Autodesk Inventor part; units mm, degrees
ref_plane "Work Plane1" through (-6.9215, -6.9215, 7.4676) normal (0, 0, -1) x (0, 1, 0)
ref_plane "YZ Plane" through (0, 0, 0) normal (1, 0, 0) x (0, 1, 0)
ref_plane "XZ Plane" through (0, 0, 0) normal (0, 1, 0) x (-1, 0, 0)
sketch "Sketch1" plane through (0, 0, 0) normal (0, 0, 1) x (1, 0, 0)
  circle A0 centre (0, 0) radius 6.477
  arc A1 (9.8184, 2.6122) -> (-9.8184, 2.6122) centre (0, 0) ccw
  line L0 (0, -10.16) -> (-20, -10.16)
  line L1 (-20, -10.16) -> (-20, -5.08)
  line L2 (0, -5.08) -> (0, -10.16)
  line L3 (0, -10.16) -> (20, -10.16)
  line L4 (20, -10.16) -> (20, -5.08)
  line L5 (0, -5.08) -> (0, -10.16)
  line L6 (-16, -5.08) -> (-16, -10.16) construction
  line L7 (-19.5, -5.08) -> (-19.5, -10.16) construction
  line L8 (-12.5, -5.08) -> (-12.5, -10.16) construction
  line L9 (-11.865, -5.08) -> (-11.865, -10.16) construction
  line L10 (-11.865, -5.08) -> (-9.8184, 2.6122)
  line L11 (16, -5.08) -> (16, -10.16) construction
  line L12 (12.5, -5.08) -> (12.5, -10.16) construction
  line L13 (11.865, -5.08) -> (11.865, -10.16) construction
  line L14 (11.865, -5.08) -> (9.8184, 2.6122)
  line L15 (20, -5.08) -> (11.865, -5.08)
  line L16 (-20, -5.08) -> (-11.865, -5.08)
  dimension "d0" = 12.954
  dimension "d1" = 20.32
  dimension "d3" = 5.08
  dimension "d5" = 5.08
  dimension "d6" = 16
  dimension "d7" = 3.5
  dimension "d8" = 3.5
  dimension "d9" = 0.635
  dimension "d10" = 16
  dimension "d11" = 3.5
  dimension "d12" = 0.635
ref_plane "Work Plane1" through (-6.9215, -6.9215, 7.4676) normal (0, 0, -1) x (0, 1, 0)
extrude "Extrusion1" add sketch "Sketch1" along normal up to surface (7.4676 mm away)
sketch "Sketch3" plane through (20, -10.16, 0) normal (1, 0, 0) x (0, 0, -1)
  line L0 (-7.4676, 5.08) -> (-7.4676, 0)
  line L1 (-7.4676, 0) -> (0, -2.5713)
  line L2 (-7.4676, 0) -> (0.6469, 0) construction
  line L3 (0, 0) -> (0, -2.5713)
  line L4 (0, 0) -> (-7.4676, 0)
  line L5 (0, 0) -> (-7.4676, 0)
  point P0 (0, 10.16)
  dimension "d28" = 19
extrude "Extrusion2" add sketch "Sketch3" against normal up to surface (40 mm away)
sketch "Sketch4" plane through (20, -5.08, 7.4676) normal (1, 0, 0) x (0, 0, -1)
  line L0 (7.4676, 0) -> (0, 0)
  line L1 (7.4676, 0) -> (0, 0)
  line L2 (7.4676, 0) -> (0, 2.5713)
  line L3 (0, 0) -> (0, 7.6922)
  line L4 (7.4676, 0) -> (15.3655, 0) construction
  line L5 (0, 7.6922) -> (0, 0)
  line L6 (0, 2.5713) -> (0, 0)
  point P0 (7.4676, 5.08)
  dimension "d31" = 161
extrude "Extrusion3" add sketch "Sketch4" against normal blind 10.16
sketch "Sketch5" plane through (-20, -5.08, 0) normal (-1, 0, 0) x (0, 0, 1)
  line L0 (7.4676, 7.6922) -> (7.4676, 0)
  line L1 (0, 0) -> (7.4676, 0)
  line L2 (0, 0) -> (7.4676, 2.5713)
  line L3 (0, 0) -> (7.8979, 0) construction
  line L4 (7.4676, 0) -> (7.4676, -5.08)
  line L5 (7.4676, 2.5713) -> (7.4676, 0)
  point P0 (0, 5.08)
  dimension "d34" = 19
extrude "Extrusion4" add sketch "Sketch5" against normal blind 10.16
sketch "Sketch6" plane through (-20, -12.7313, 0) normal (0, -0.9455, 0.3256) x (1, 0, 0)
  line L0 (40, 2.491) -> (40, 10.3889) construction
  line L1 (40, 3.8979) -> (0, 3.8979) construction
  line L2 (0, 7.8979) -> (40, 7.8979) construction
  line L3 (36, 7.8979) -> (36, 0) construction
  line L4 (40, 0) -> (0, 0) construction
  line L5 (40, 7.8979) -> (40, 0) construction
  line L6 (4, 7.8979) -> (4, 0) construction
  line L7 (0, 7.8979) -> (0, 0) construction
  circle A0 centre (36, 3.8979) radius 2.1844
  circle A1 centre (4, 3.8979) radius 2.1844
  point P0 (20, 4.1449)
  dimension "d37" = 4
  dimension "d38" = 4
  dimension "d39" = 4
  dimension "d40" = 4.3688
  dimension "d41" = 4.3688
hole "Hole2" at (16, -11.4623, 3.6855) at (-16, -11.4623, 3.6855) direction (0, 0.9455, -0.3256) diameter 4.3688 end through all
properties part number "omni wheel shaft holder low channel side attach"
Check sheet for the modelled part. Datum: model origin and axes. Units: mm. A direction names the side the tool comes from. Coordinates: 2 decimals unless noted, no trailing zeros. Loops run counter-clockwise (first coordinate to the right, second up) from the corner with the lowest first, then second, coordinate; pieces in that order, holes last.
1) Access from +Z, -Z, +X, -X, +Y, -Y to the whole of each face (thin tool, end or side, straight path). Record for faces 5 (the face through (0, -7, 7.468)), 6 (the face through (-10.629, -0.433, 3.682)), 7 (the face through (15.652, -3.527, 4.511)).
2) Sectioned sample at C-C (z = 6.75). Record the boundary of the cut face in (x, y).
3) Sectioned sample at D-D (z = 2). Count the separate pieces of the cut face and the enclosed holes in it, and give its area (3 significant figures).
4) Sectioned sample at B-B (y = -3.25). Record the boundary of the cut face in (x, z), and give its area (3 significant figures).
5) Release check for a two-part mould opening along Y. For faces 1 (the face through (-20, -8, 4)), 2 (the face through (-0.19, 10.16, 3.68)), 3 (the face through (0.28, -11.428, 3.786)), 4 (the face through (-16.096, -7.284, 4.555)) record: released by +Y, released by -Y, zero draft, split by the parting line, or undercut.
6) Gauge pin test, flat ends, axial feed: pin 1 (1 mm diameter, centred on x = -2, z = 3.5, fed in from +Y); pin 2 (3 mm diameter, centred on x = 7.5, z = 4, fed in from +Y). Record the tip position at first contact, or that the pin passes through.
7) Material ranges on probe 1 along Y at (x, z) = (-3, 6.25); probe 2 along X at (y, z) = (-5.5, 5); probe 3 along X at (y, z) = (4, 5.25), recorded low to high.
8) Sectioned sample at A-A (x = 0). Record the boundary of the cut face in (y, z).
Check sheet entries:
1. face 5: +Z, +X, -X, +Y, -Y
1. face 6: -Z, -X, +Y
1. face 7: -Z, +X, +Y
2. outline: (-20, -10.41) - (20, -10.41) - (20, -2.76) - (11.25, -2.76) - (9.82, 2.61) arc R10.16 ccw to (-9.82, 2.61) - (-11.25, -2.76) - (-20, -2.76) - close; hole circle Ø12.95 at (0, 0)
3. separate pieces: 3
3. enclosed holes: 1
3. area: 374 mm2
4. outline: (-20, 5.31) - (-11.38, 5.31) - (-11.38, 0) - (-5.6, 0) - (-5.6, 7.47) - (-20, 7.47) - close; (5.6, 0) - (11.38, 0) - (11.38, 5.31) - (20, 5.31) - (20, 7.47) - (5.6, 7.47) - close
4. area: 123 mm2
5. face 1: zero draft
5. face 2: released by +Y
5. face 3: released by -Y
5. face 4: undercut
6. pin 1: stops at y = 10.05
6. pin 2: stops at y = 8.2
7. probe 1: y = -10.58 to -5.74, 5.74 to 9.71
7. probe 2: x = -20 to -3.42, 3.42 to 20
7. probe 3: x = -9.34 to -5.09, 5.09 to 9.34
8. outline: (-12.73, 0) - (-6.48, 0) - (-6.48, 7.47) - (-10.16, 7.47) - close; (6.48, 0) - (10.16, 0) - (10.16, 7.47) - (6.48, 7.47) - close
